Source: CAD feature listing. Evaluate the final solid. Frame: model axes, mm. Face numbers are marked on the shaded views. Round coordinates to 2 decimals unless told otherwise and drop trailing zeros. Order: outer loops, then holes, each group sorted by start corner. A loop starts at its lowest first (then second) coordinate and runs counter-clockwise, first axis right, second up. Notation, with made-up numbers: (55.25, 76.5) -> (83.25, 76.5) arc R20 ccw to (83.25, 102.5) -> close; hole circle Ø6 at (23, -11.75). An arc over 180 degrees is marked (long way). Write item = value, one per line. Start each with the question number.
(1) Contact query for flat-ended pins moving along their axis: pin 1 Ø8 at (x, y) = (2.5, -2.5) entering from -Z; pin 2 Ø0.9 at (x, z) = (-0.5, -0.5) entering from +Y; pin 3 Ø2 at (x, z) = (6, 0.5) entering from +Y; pin 4 Ø6 at (x, y) = (0.5, 1) entering from +Z. Output: stop coordinate, or through.
(2) Cut plane B-B on y = -10.5. Return the cut outline in (x, z), then the cut area to 3 significant figures.
(3) Cut plane A-A on x = 0. Return the cut outline in (y, z), then the cut area to 3 significant figures.
(4) Draft query along Y for the marked faces 1, 2, 3 and 4. Return one class per face: released by +Y, released by -Y, zero draft, split by the parting line, or undercut.
(5) Ray query, line 1 (Z direction, x = -5.25, y = -4.25); line 2 (X direction, y = 1.5, z = 0.5); line 3 (X direction, y = -2, z = -1). Return the intervals inside material, ascending.
from build123d import *
from build123d.topology import SkipClean

# Parameters (mm, degrees)
ESQUISSE2_R        = 1.75
BOSS_EXTRU_1_START = -8.5
ESQUISSE3_R        = 3
BOSS_EXTRU_1_DEPTH = 4
BOSS_EXTRU_1_TAPER = 20
ESQUISSE4_R        = 2
BOSS_EXTRU_2_DEPTH = 10


with BuildPart() as part:
    # Esquisse2 → Révolution1 (revolve)
    with BuildSketch(Plane(origin=(0, 0, 0), x_dir=(1, 0, 0), z_dir=(0, 1, 0))):
        with Locations((6.75, 0)):
            Circle(ESQUISSE2_R)
    revolve(axis=Axis((0, 0, 0), (0, 0, -1)))



with BuildPart() as body_2:
    # Esquisse3 → Boss.-Extru.1 (new body)
    with BuildSketch(Plane(origin=(0, 0, 0), x_dir=(1, 0, 0), z_dir=(0, 1, 0)).offset(BOSS_EXTRU_1_START)):
        Circle(ESQUISSE3_R)
    extrude(amount=BOSS_EXTRU_1_DEPTH, taper=BOSS_EXTRU_1_TAPER)


with BuildPart() as part_1:
    with SkipClean():  # the faces are left unmerged after this step: merging them gives an invalid solid
        add(part.part)

        add(body_2.part)  # Boss.-Extru.2 merges body 2
        # Esquisse4 → Boss.-Extru.2 (add)
        with BuildSketch(Plane.XZ.offset(8.5)):
            with Locations(Location((0, 0, 0), (0, 0, 270))):
                Circle(ESQUISSE4_R)
        extrude(amount=BOSS_EXTRU_2_DEPTH)


solid = part_1.part
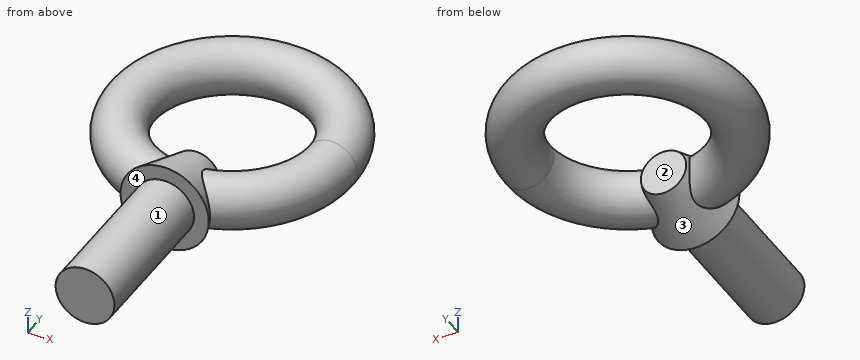
Evaluation:
q1.pin_1 = -2.02
q1.pin_2 = 8.49
q1.pin_3 = 6.83
q1.pin_4 = through
q2.outline = circle Ø4 at (0, 0)
q2.area = 12.6 mm^2
q3.outline = (-18.5, -2) -> (-8.5, -2) -> (-8.5, -3) -> (-4.5, -1.54) -> (-4.5, 1.54) -> (-8.5, 3) -> (-8.5, 2) -> (-18.5, 2) -> close; circle Ø3.5 at (6.75, 0)
q3.area = 67.8 mm^2
q4.face_1 = zero draft
q4.face_2 = undercut
q4.face_3 = undercut
q4.face_4 = released by -Y
q5.line_1 = -1.75 to 1.75
q5.line_2 = -8.29 to -4.85, 4.85 to 8.29
q5.line_3 = -7.94 to -4.92, 4.92 to 7.94
